Here's how the part is built. I have some questions about the finished solid (model axes, mm). A direction names the side the tool comes from. Give positions to 0.01 mm unless a question says otherwise; leave off trailing zeros. Write each loop counter-clockwise with the first axis right and the second up, starting at its lowest first coordinate (ties: lowest second). Pieces come first, ordered by that corner, then holes. Notation, with made-up numbers: (6, -8.75) -> (25, -8.75) arc R23 ccw to (25, 18.25) -> close; hole circle Ø8 at (-8.5, 20.5). An arc over 180 degrees is marked (long way). Use CSV: the item, a comma, the result in double quotes. Start each with the question number.
(1) Suppose I cut it at A-A on y = 1. List the corners of the cut face in (x, z) for me.
(2) Suppose I cut it at B-B on y = 6.75. List the corners of the cut face in (x, z) for me, plus the area to 3 significant figures.
(3) For pin 1 Ø12 at (x, z) = (34, -19) entering from +Y; pin 2 Ø4.5 at (y, z) = (5.5, -42) entering from +X; pin 3 Ø3 at (x, z) = (19, -40) entering from +Y; pin 4 Ø4.5 at (y, z) = (3.5, -44) entering from -X, each with a flat end and sliding along its axis, tell me the tip position at first contact or that it passes through.
(4) I need wall thicknesses on L1, parallel to X at y = 3.25, z = -42; L2, parallel to X at y = 6, z = -51; L3, parallel to X at y = 4.75, z = -17.5. Which ranges of each line are inside material? Lowest first, please. Write a range as [from, to].
(5) Which directions (+Z, -Z, +X, -X, +Y, -Y) give clear straight access to the entire face, cutting with the end or side of a thin tool? Please do faces 1 (the cylindrical face through (29.25, 4.44, -31.43)), 2 (the flat face through (19.25, 3, -41)), 3 (the cylindrical face through (17.7, 7, -55.8)), 4 (the flat face through (5, 5, -21)).
(6) If we mould it in two halves opening along X, with no side actions, what happens to faces 5 (the flat face through (7.75, 5, -47)), 6 (the flat face through (70.5, 5, -21)), 7 (the flat face through (60.55, 7, -41))? For each: pulls with the +X half, pulls with the -X half, needs draft (parallel to the pull), parting line crosses it, or undercut.
from build123d import *

# Parameters (mm, degrees)
BOSS_EXTRUDE1_DEPTH = 9
CUT_EXTRUDE2_REACH  = 98.857
SKETCH5_W           = 20
SKETCH5_H           = 30
SKETCH5_W_2         = 7.75
CUT_EXTRUDE3_DEPTH  = 10
FILLET1_R           = 5
CUT_EXTRUDE4_DEPTH  = 4
CHAMFER1_SIZE       = 9
CHAMFER1_SIZE_2     = 4.196768923
CUT_EXTRUDE5_REACH  = 98.857
SKETCH7_W           = 5
SKETCH7_H           = 33.085129134
SKETCH7_H_2         = 33.745309592


with BuildPart() as part:
    # Sketch1 → Boss-Extrude1 (new body)
    with BuildSketch(Plane(origin=(0, 0, 0), x_dir=(1, 0, 0), z_dir=(0, 1, 0))):
        with BuildLine():
            Line((0, 0), (0, 60))
            Line((0, 60), (75.5, 60))
            Line((75.5, 60), (75.5, 0))
            ThreePointArc((75.5, 0), (37.75, 20.506378381), (0, 0))
        make_face()
    extrude(amount=BOSS_EXTRUDE1_DEPTH)

    # Sketch4 → Cut-Extrude2 (cut, up to next)
    with BuildSketch(Plane(origin=(0, 9, 0), x_dir=(1, 0, 0), z_dir=(0, 1, 0)), mode=Mode.PRIVATE) as cut_extrude2_sk1:
        with BuildLine():
            Line((19.25, 53), (19.25, 28))
            ThreePointArc((19.25, 28), (17.75, 26.5), (16.25, 28))
            Line((16.25, 28), (16.25, 53))
            ThreePointArc((16.25, 53), (17.75, 54.5), (19.25, 53))
        make_face()
    cut_extrude2_tool1 = extrude(cut_extrude2_sk1.sketch, amount=-CUT_EXTRUDE2_REACH, mode=Mode.PRIVATE) & part.part
    # Sketch4 → Cut-Extrude2 (cut, up to next)
    with BuildSketch(Plane(origin=(0, 9, 0), x_dir=(1, 0, 0), z_dir=(0, 1, 0)), mode=Mode.PRIVATE) as cut_extrude2_sk2:
        with BuildLine():
            Line((59.25, 53), (59.25, 28))
            ThreePointArc((59.25, 28), (57.75, 26.5), (56.25, 28))
            Line((56.25, 28), (56.25, 53))
            ThreePointArc((56.25, 53), (57.75, 54.5), (59.25, 53))
        make_face()
    cut_extrude2_tool2 = extrude(cut_extrude2_sk2.sketch, amount=-CUT_EXTRUDE2_REACH, mode=Mode.PRIVATE) & part.part
    add(cut_extrude2_tool1.solids().sort_by_distance((17.75, 9, -40.5))[0], mode=Mode.SUBTRACT)
    add(cut_extrude2_tool2.solids().sort_by_distance((57.75, 9, -40.5))[0], mode=Mode.SUBTRACT)

    # Sketch5 → Cut-Extrude3 (cut)
    with BuildSketch(Plane(origin=(0, 9, 0), x_dir=(1, 0, 0), z_dir=(0, 1, 0))):
        with Locations((37.75, 45)):
            Rectangle(SKETCH5_W, SKETCH5_H)
        with Locations((71.625, 45)):
            Rectangle(SKETCH5_W_2, SKETCH5_H)
        with Locations((3.875, 45)):
            Rectangle(SKETCH5_W_2, SKETCH5_H)
    extrude(amount=-CUT_EXTRUDE3_DEPTH, mode=Mode.SUBTRACT)

    # Fillet1
    fillet1_edges = [part.edges().sort_by_distance(p)[0] for p in [
        (27.75, 4.5, -30),
        (47.75, 4.5, -30),
        (7.75, 4.5, -30),
        (67.75, 4.5, -30),
    ]]
    fillet(fillet1_edges, radius=FILLET1_R)

    # Sketch6 → Cut-Extrude4 (cut)
    with BuildSketch(Plane(origin=(0, 9, 0), x_dir=(1, 0, 0), z_dir=(0, 1, 0))):
        with BuildLine():
            Line((20.55, 53), (20.55, 28))
            ThreePointArc((20.55, 28), (17.75, 25.2), (14.95, 28))
            Line((14.95, 28), (14.95, 53))
            ThreePointArc((14.95, 53), (17.75, 55.8), (20.55, 53))
        make_face()
        with BuildLine():
            Line((60.55, 53), (60.55, 28))
            ThreePointArc((60.55, 28), (57.75, 25.2), (54.95, 28))
            Line((54.95, 28), (54.95, 53))
            ThreePointArc((54.95, 53), (57.75, 55.8), (60.55, 53))
        make_face()
    extrude(amount=-CUT_EXTRUDE4_DEPTH, mode=Mode.SUBTRACT)

    # Chamfer1
    # the kernel refuses this chamfer: 9, 4.196768923 mm, written as the material it takes off along each edge
    with BuildSketch(Plane(origin=(37.75, 9, 24.493621619), x_dir=(0.9983743289729347, 0, -0.05699736176212511), z_dir=(0.05699736176212511, 0, 0.9983743289729347))) as chamfer1_piece_1:
        Polygon((45, -CHAMFER1_SIZE), (45 + CHAMFER1_SIZE_2, 0), (45, 0), align=None)
    revolve(axis=Axis((37.75, 9, 24.493621619), (0, 1, 0)), revolution_arc=173.465041841, mode=Mode.SUBTRACT)

    # Sketch7 → Cut-Extrude5 (cut, up to next)
    with BuildSketch(Plane(origin=(0, 9, 0), x_dir=(1, 0, 0), z_dir=(0, 1, 0)), mode=Mode.PRIVATE) as cut_extrude5_sk1:
        with Locations((2.5, 16.542564567)):
            Rectangle(SKETCH7_W, SKETCH7_H)
    cut_extrude5_tool1 = extrude(cut_extrude5_sk1.sketch, amount=-CUT_EXTRUDE5_REACH, mode=Mode.PRIVATE) & part.part
    # Sketch7 → Cut-Extrude5 (cut, up to next)
    with BuildSketch(Plane(origin=(0, 9, 0), x_dir=(1, 0, 0), z_dir=(0, 1, 0)), mode=Mode.PRIVATE) as cut_extrude5_sk2:
        with Locations((73, 16.872654796)):
            Rectangle(SKETCH7_W, SKETCH7_H_2)
    cut_extrude5_tool2 = extrude(cut_extrude5_sk2.sketch, amount=-CUT_EXTRUDE5_REACH, mode=Mode.PRIVATE) & part.part
    add(cut_extrude5_tool1.solids().sort_by_distance((2.5, 9, -16.542565))[0], mode=Mode.SUBTRACT)
    add(cut_extrude5_tool2.solids().sort_by_distance((73, 9, -16.872655))[0], mode=Mode.SUBTRACT)


solid = part.part
Geometry says:
1,outline,"(5, -30.53) arc R5 cw to (7.75, -35) -> (7.75, -60) -> (27.75, -60) -> (27.75, -35) arc R5 cw to (32.75, -30) -> (42.75, -30) arc R5 cw to (47.75, -35) -> (47.75, -60) -> (67.75, -60) -> (67.75, -35) arc R5 cw to (70.5, -30.53) -> (70.5, -7.04) arc R45.47 cw to (5, -7.04) -> close; hole (16.25, -53) arc R1.5 ccw to (19.25, -53) -> (19.25, -28) arc R1.5 ccw to (16.25, -28) -> close; hole (56.25, -53) arc R1.5 ccw to (59.25, -53) -> (59.25, -28) arc R1.5 ccw to (56.25, -28) -> close"
2,outline,"(5, -30.53) arc R5 cw to (7.75, -35) -> (7.75, -60) -> (27.75, -60) -> (27.75, -35) arc R5 cw to (32.75, -30) -> (42.75, -30) arc R5 cw to (47.75, -35) -> (47.75, -60) -> (67.75, -60) -> (67.75, -35) arc R5 cw to (70.5, -30.53) -> (70.5, -10.8) arc R48.15 cw to (5, -10.8) -> close; hole (14.95, -53) arc R2.8 ccw to (20.55, -53) -> (20.55, -28) arc R2.8 ccw to (14.95, -28) -> close; hole (54.95, -53) arc R2.8 ccw to (60.55, -53) -> (60.55, -28) arc R2.8 ccw to (54.95, -28) -> close"
2,area,"1,570 mm²"
3,pin 1,"y = 9"
3,pin 2,"x = 67.75"
3,pin 3,"y = 5"
3,pin 4,"x = 7.75"
4,L1,"[7.75, 16.25], [19.25, 27.75], [47.75, 56.25], [59.25, 67.75]"
4,L2,"[7.75, 14.95], [20.55, 27.75], [47.75, 54.95], [60.55, 67.75]"
4,L3,"[5, 16.17], [59.33, 70.5]"
5,face 1,"-Z, +Y, -Y"
5,face 2,"+Y, -Y"
5,face 3,"+Y"
5,face 4,"+Z, -Z, -X, +Y, -Y"
6,face 5,"pulls with the -X half"
6,face 6,"pulls with the +X half"
6,face 7,"undercut"
